Here's how the part is built. I have some questions about the finished solid (model axes, mm). A direction names the side the tool comes from. Give positions to 0.01 mm unless a question says otherwise; leave off trailing zeros. Write each loop counter-clockwise with the first axis right and the second up, starting at its lowest first coordinate (ties: lowest second). Pieces come first, ordered by that corner, then holes. Notation, with made-up numbers: (55, 7.5) - (107, 7.5) arc R21 ccw to (107, 29.5) - close; hole circle Ø8 at (79, 14.25). An arc over 180 degrees is marked (long way). Use a Markdown table: item, result.
```python
from build123d import *

# Parameters (mm, degrees)
SKETCH_R           = 4
PAD_DEPTH          = 20
SKETCH001_R        = 6.2
POCKET_DEPTH       = 15
SKETCH002_R        = 2.25
POCKET001_DEPTH    = 69
POLARPATTERN_COUNT = 2
POLARPATTERN_ANGLE = 120


with BuildPart() as part:
    # Sketch → Pad (new body)
    with BuildSketch(Plane.XY):
        with BuildLine():
            ThreePointArc((7.5, -19.615045), (0, 21), (-7.5, -19.615045))
            Line((-7.5, -19.615045), (7.5, -19.615045))
        make_face()
        Circle(SKETCH_R, mode=Mode.SUBTRACT)
    extrude(amount=PAD_DEPTH)

    # Sketch001 (on DatumPlane) → Pocket (cut)
    with BuildSketch(Plane.XZ.offset(19.615045)):
        with Locations((0, 10)):
            Circle(SKETCH001_R)
    extrude(amount=-POCKET_DEPTH, mode=Mode.SUBTRACT)

    # Sketch002 (on DatumPlane) → Pocket001 (cut)
    with BuildSketch(Plane(origin=(0, 0, 10), x_dir=(0.5, -0.866025, 0), z_dir=(0.866025, 0.5, 0))):
        Circle(SKETCH002_R)
    pocket001 = extrude(amount=POCKET001_DEPTH, mode=Mode.SUBTRACT)

    # PolarPattern: Pocket001 ×2 about axis
    polarpattern_axis = Axis((0, 0, 0), (0, 0, 1))
    for i in range(1, POLARPATTERN_COUNT):
        add(pocket001.rotate(polarpattern_axis, i * POLARPATTERN_ANGLE / (POLARPATTERN_COUNT - 1)), mode=Mode.SUBTRACT)


solid = part.part
```
Item 1: Thinking about a two-plate mould opening in X: for faces 1 (the cylindrical face through (-10.57, 5.76, 7.77)), 2 (the flat face through (4.4, 1, 0)), 3 (the cylindrical face through (0.816, 20.984, 9.86)), which applies, +X half, -X half, draft (parallel to the pull), parting line (faces both ways), or undercut?
Values:
| item | result |
|---|---|
| face 1 | undercut |
| face 2 | draft |
| face 3 | parting line |
Item 2: If we section it at B-B, the plane z = 11.75: Write out the boundary of the cut face in (x, y), plus the area to 3 significant figures.
Values:
| item | result |
|---|---|
| outline | (-18.85, 9.25) arc R21 ccw to (-7.5, -19.62) - (-5.95, -19.62) - (-5.95, -4.62) - (5.95, -4.62) - (5.95, -19.62) - (7.5, -19.62) arc R21 ccw to (18.85, 9.25) - (3.95, 0.65) arc R4 cw (long way) to (-3.95, 0.65) - close; (-17.44, 11.7) - (-2.53, 3.1) arc R4 cw to (2.53, 3.1) - (17.44, 11.7) arc R21 ccw to start |
| area | 1,050 mm2 |
Item 3: I need wall thicknesses on line 1 along Z through (x, y) = (0, -16); line 2 along Y through (x, z) = (11.5, 10.75); line 3 along X through (y, z) = (-5.5, 7.5). Which ranges of each line are inside material? Lowest first, please. Write a range as [from, to].
Values:
| item | result |
|---|---|
| line 1 | z = [0, 3.8], [16.2, 20] |
| line 2 | y = [-17.57, 4.19], [9.09, 17.57] |
| line 3 | x = [-20.27, -5.67], [5.67, 20.27] |
Item 4: If we section it at C-C, the plane z = 18: Write out the boundary of the cut face in (x, y).
Values:
| item | result |
|---|---|
| outline | (-7.5, -19.62) - (7.5, -19.62) arc R21 ccw (long way) to start; hole circle Ø8 at (0, 0) |
Item 5: For faces 4 (the flat face through (0, -19.615, 3)), 5 (the flat face through (0, -4.615, 10)), which set-ups out of +Z, -Z, +X, -X, +Y, -Y let a thin tool reach every point of the face, with its end or its side?
Values:
| item | result |
|---|---|
| face 4 | +Z, -Z, +X, -X, -Y |
| face 5 | -Y |
Item 6: If we section it at A-A, the plane x = 0: Write out the boundary of the cut face in (y, z).
Values:
| item | result |
|---|---|
| outline | (-19.62, 0) - (-4, 0) - (-4, 20) - (-19.62, 20) - (-19.62, 16.2) - (-4.62, 16.2) - (-4.62, 3.8) - (-19.62, 3.8) - close; (4, 0) - (21, 0) - (21, 20) - (4, 20) - close |
Item 7: If we section it at D-D, the plane y = -10.5: Write out the boundary of the cut face in (x, z).
Values:
| item | result |
|---|---|
| outline | (-18.19, 0) - (18.19, 0) - (18.19, 20) - (-18.19, 20) - close; hole circle Ø12.4 at (0, 10) |
Item 8: Will these pins go through, and if not, where does the flat tip stop? pin 1 Ø10 at (x, z) = (-0.5, 11) entering from -Y; pin 2 Ø8 at (y, z) = (-13.5, 7.5) entering from -X; pin 3 Ø1.5 at (y, z) = (9.5, 3.5) entering from -X; pin 4 Ø10.5 at (x, y) = (0, 0) entering from -Z.
Values:
| item | result |
|---|---|
| pin 1 | stops at y = -4.62 |
| pin 2 | stops at x = -18.73 |
| pin 3 | stops at x = -19.09 |
| pin 4 | stops at z = 0 |
